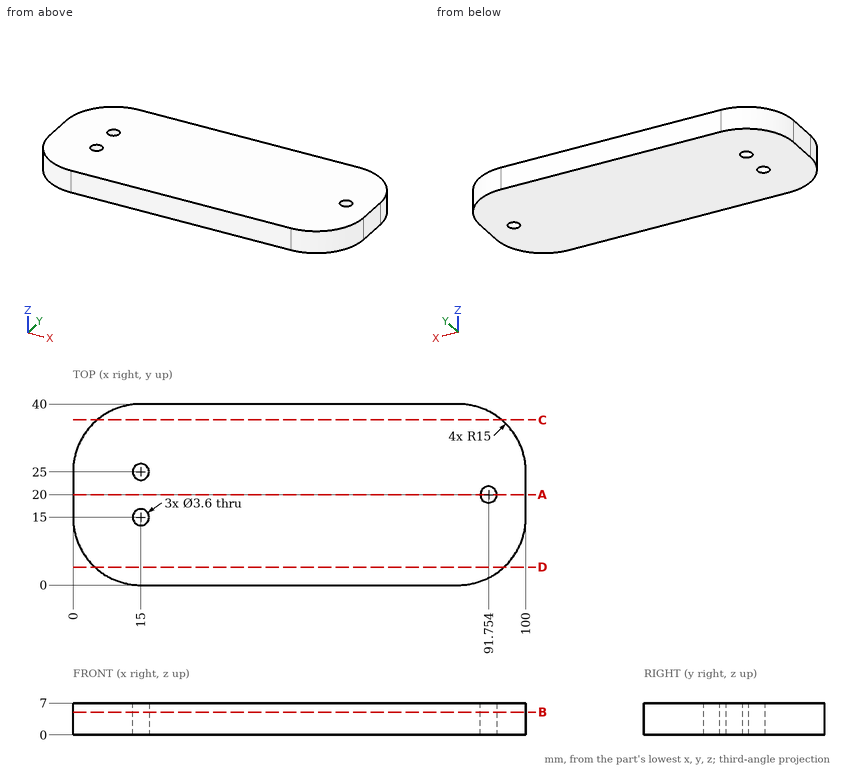
Job drawing, mm, ordinate dimensions from the low corner. One solid piece. Round coordinates to 2 decimals unless told otherwise and drop trailing zeros. Write each loop counter-clockwise with the first axis right and the second up, starting at its lowest first coordinate (ties: lowest second). Pieces come first, ordered by that corner, then holes. Notation, with made-up numbers: M 86.25,21 L 127.25,21 A22 cw 127.25,49 Z; hole C 47.5,-1 d9. An arc over 180 degrees is marked long. Return JSON: item names as keys, results as strings. Group by question number.
(1) Saw through at D-D on y = 4. Write the cut outline in (x, z).
(2) Saw through at C-C on y = 36.5. Write the cut outline in (x, z), then the cut area to 3 significant figures.
(3) Saw through at B-B on z = 5. Write the cut outline in (x, y).
(4) Saw through at A-A on y = 20. Write the cut outline in (x, z), then the cut area to 3 significant figures.
(5) Drill centre lines: probe 1 along X at (y, z) = (24, 4.75); probe 2 along X at (y, z) = (19.5, 2.25) (1 decimal); probe 3 along Y at (x, z) = (10, 5.75). Where is each one in solid material? Low to high.
Returned:
{
 "1": {"outline": "M 4.8,0 L 95.2,0 L 95.2,7 L 4.8,7 Z"},
 "2": {"outline": "M 5.37,0 L 94.63,0 L 94.63,7 L 5.37,7 Z", "area": "625 mm²"},
 "3": {"outline": "M 0,15 A15 ccw 15,0 L 85,0 A15 ccw 100,15 L 100,25 A15 ccw 85,40 L 15,40 A15 ccw 0,25 Z; hole C 15,15 d3.6; hole C 15,25 d3.6; hole C 91.75,20 d3.6"},
 "4": {"outline": "M 0,0 L 89.95,0 L 89.95,7 L 0,7 Z; M 93.55,0 L 100,0 L 100,7 L 93.55,7 Z", "area": "675 mm²"},
 "5": {"probe 1": "0 to 13.5, 16.5 to 100", "probe 2": "0 to 90, 93.5 to 100", "probe 3": "0.86 to 39.14"}
}
